Input: part model. Units: mm. Frame: model coordinates. A direction names the side the tool comes from. Coordinates: 2 decimals unless noted, no trailing zeros. Order: outer loops, then holes, each group sorted by start corner. A loop starts at its lowest first (then second) coordinate and runs counter-clockwise, first axis right, second up. Notation, with made-up numbers: (46, 58.5) -> (89, 58.5) arc R16 cw to (89, 62.5) -> close; hole circle Ø8 at (85.25, 31.25). An arc over 180 degrees is marked (long way). Use one line per item in the form item = value. Start each with the question number.
1) Pin query (flat end, axial travel): pin 1 (0.5 mm diameter, centred on y = 5, z = -2.5, fed in from -X); pin 2 (2.5 mm diameter, centred on x = 2, y = 5, fed in from +Z); pin 3 (1.5 mm diameter, centred on x = -2.5, y = 4.5, fed in from -Z). Return the tip coordinate at first contact, or that it passes through.
2) Section query D-D on z = -2.5. Output: boundary loops of the cut face in (x, y), then the cut area to 3 significant figures.
3) Access query for faces 4 (the flat face through (-0.1, 0, 0.3)), 5 (the cylindrical face through (-1.42, 8.28, -2.15)), 6 (the flat face through (4, 8, -1.027)). Directions: +Z, -Z, +X, -X, +Y, -Y. A direction counts if a zero-diameter tool reaches every point of the face in a straight line with its end or side. Return the directions, or none.
4) Ray query, line 1 along Z through (x, y) = (3.5, 1.5); line 2 along X through (y, z) = (13.25, 0); line 3 along X through (y, z) = (7, -2.5). Return the intervals inside material, ascending.
5) Section query C-C on y = 7. Output: boundary loops of the cut face in (x, z), then the cut area to 3 significant figures.
6) Section query B-B on z = -1.5. Output: boundary loops of the cut face in (x, y), then the cut area to 3 significant figures.
7) Draft query along X for faces 1 (the flat face through (4.535, 8, -3)), 2 (the flat face through (-0.1, 16.8, 0.3)), 3 (the flat face through (2, 8, -3.027)). Return one class per face: pulls with the +X half, pulls with the -X half, needs draft (parallel to the pull), parting line crosses it, or undercut.
8) Section query A-A on y = 10.75. Output: boundary loops of the cut face in (x, z), then the cut area to 3 significant figures.
from build123d import *

# Parameters (mm, degrees)
BOSS_EXTRUDE1_DEPTH = 16.8
SKETCH3_R           = 1.602221917
CUT_EXTRUDE2_DEPTH  = 1


with BuildPart() as part:
    # Sketch1 → Boss-Extrude1 (new body)
    with BuildSketch(Plane(origin=(0, 0, 0), x_dir=(1, 0, 0), z_dir=(0, 1, 0))):
        with BuildLine():
            Line((-4.627081214, -3.973073539), (-1.569860328, -3.973073539))
            ThreePointArc((-1.569860328, -3.973073539), (-1.400678587, -3.120671939), (-1.229309949, -2.268707303))
            Line((-1.229309949, -2.268707303), (2.8066913, 1.026926461))
            Line((2.8066913, 1.026926461), (4.535241357, 1.026926461))
            Line((4.535241357, 1.026926461), (4.535241357, 4.026926461))
            Line((4.535241357, 4.026926461), (1.078141243, 4.026926461))
            ThreePointArc((1.078141243, 4.026926461), (-2.077248816, 2.905523317), (-3.817253142, 0.044331891))
            ThreePointArc((-3.817253142, 0.044331891), (-4.228191177, -1.963156507), (-4.627081214, -3.973073539))
        make_face()
        with BuildLine():
            Line((-3.410627534, -2.973073539), (-2.390949988, -2.973073539))
            ThreePointArc((-2.390949988, -2.973073539), (-2.265209784, -2.346372679), (-2.138290376, -1.719909567))
            Line((-2.138290376, -1.719909567), (2.450276186, 2.026926461))
            Line((2.450276186, 2.026926461), (3.535241357, 2.026926461))
            Line((3.535241357, 2.026926461), (3.535241357, 3.026926461))
            Line((3.535241357, 3.026926461), (1.078141243, 3.026926461))
            ThreePointArc((1.078141243, 3.026926461), (-1.446170804, 2.129803946), (-2.838174265, -0.159149195))
            ThreePointArc((-2.838174265, -0.159149195), (-3.127366046, -1.56550815), (-3.410627534, -2.973073539))
        make_face(mode=Mode.SUBTRACT)
    extrude(amount=BOSS_EXTRUDE1_DEPTH)

    # Sketch3 → Cut-Extrude2 (cut)
    with BuildSketch(Plane(origin=(0.619682886, 0, 0.758895279), x_dir=(0.774572925, 0, -0.632484612), z_dir=(0.632484612, 0, 0.774572925))):
        with Locations((0.218194806, 8.4)):
            Circle(SKETCH3_R)
    extrude(amount=-CUT_EXTRUDE2_DEPTH, mode=Mode.SUBTRACT)


solid = part.part
Answers below:
q1.pin_1 = -2.74
q1.pin_2 = 0.65
q1.pin_3 = -3.15
q2.outline = (-2.52, 0) -> (-0.91, 0) -> (-0.91, 16.8) -> (-2.52, 16.8) -> close; (3.54, 0) -> (4.54, 0) -> (4.54, 16.8) -> (3.54, 16.8) -> close
q2.area = 43.9 mm^2
q3.face_4 = +Z, -Z, +X, -X, -Y
q3.face_5 = +Y, -Y
q3.face_6 = +Z, +X, +Y, -Y
q4.line_1 = -4.03 to -3.03, -2.03 to -1.03
q4.line_2 = -3.83 to -2.8, -0.03 to 1.55
q4.line_3 = -2.52 to -0.91, 3.54 to 4.54
q5.outline = (-4.63, 3.97) arc R341.64 ccw to (-3.82, -0.04) arc R5 ccw to (1.08, -4.03) -> (4.54, -4.03) -> (4.54, -1.03) -> (2.81, -1.03) -> (1.39, 0.13) -> (0.76, -0.65) -> (2.45, -2.03) -> (3.54, -2.03) -> (3.54, -3.03) -> (1.08, -3.03) arc R4 cw to (-2.84, 0.16) arc R340.64 cw to (-3.41, 2.97) -> (-2.39, 2.97) arc R339.64 ccw to (-2.14, 1.72) -> (-0.45, 0.34) -> (0.19, 1.11) -> (-1.23, 2.27) arc R338.64 cw to (-1.57, 3.97) -> close
q5.area = 23.6 mm^2
q6.outline = (-3.27, 0) -> (-2.07, 0) -> (-2.07, 16.8) -> (-3.27, 16.8) -> close; (1.8, 0) -> (4.54, 0) -> (4.54, 16.8) -> (1.8, 16.8) -> close
q6.area = 66.1 mm^2
q7.face_1 = pulls with the +X half
q7.face_2 = needs draft
q7.face_3 = undercut
q8.outline = (-4.63, 3.97) arc R341.64 ccw to (-3.82, -0.04) arc R5 ccw to (1.08, -4.03) -> (4.54, -4.03) -> (4.54, -1.03) -> (2.81, -1.03) -> (-1.23, 2.27) arc R338.64 cw to (-1.57, 3.97) -> close; hole (-3.41, 2.97) arc R340.64 ccw to (-2.84, 0.16) arc R4 ccw to (1.08, -3.03) -> (3.54, -3.03) -> (3.54, -2.03) -> (2.45, -2.03) -> (-2.14, 1.72) arc R339.64 cw to (-2.39, 2.97) -> close
q8.area = 25.1 mm^2
